```python
from build123d import *

# Parameters (mm, degrees)
F1_DEPTH = 25.4
F3_D     = 3.7973
F3_DEPTH = 101.6
F3_TIP   = 1.1408240143
F4_R     = 2.54


with BuildPart() as f1:
    # F0 (on Front) → F1 (new body)
    with BuildSketch(Plane.XZ):
        with BuildLine():
            ThreePointArc((11.684, 0), (0, -11.684), (-11.684, 0))
            Line((-11.684, 0), (-11.684, 11.684))
            Line((-11.684, 11.684), (-31.75, 11.684))
            Line((-31.75, 11.684), (-31.75, 6.604))
            Line((-31.75, 6.604), (-16.764, 6.604))
            Line((-16.764, 6.604), (-16.764, 0))
            ThreePointArc((-16.764, 0), (0, -16.764), (16.764, 0))
            Line((16.764, 0), (16.764, 6.604))
            Line((16.764, 6.604), (31.75, 6.604))
            Line((31.75, 6.604), (31.75, 11.684))
            Line((31.75, 11.684), (11.684, 11.684))
            Line((11.684, 11.684), (11.684, 0))
        make_face()
    extrude(amount=F1_DEPTH)

    # F3
    with Locations(Plane(origin=(0, 0, 6.604), x_dir=(1, 0, 0), z_dir=(0, 0, -1))):
        with Locations((-25.4, 12.7), (25.4, 12.7)):
            Hole(F3_D / 2, depth=F3_DEPTH)
            with Locations((0, 0, -(F3_DEPTH + F3_TIP / 2))):  # 118° drill point
                Cone(0, F3_D / 2, F3_TIP, mode=Mode.SUBTRACT)

    # F4
    f4_edges = [f1.edges().sort_by_distance(p)[0] for p in [
        (16.764, -12.7, 6.604),
        (-16.764, -12.7, 6.604),
    ]]
    fillet(f4_edges, radius=F4_R)


solid = f1.part
```
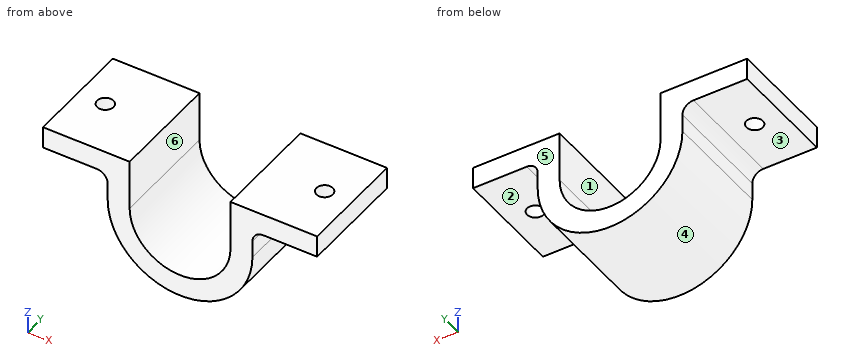
Geometry check sheet. Reference: the model listing, model coordinates, mm. Face numbers are marked on the shaded views. A direction names the side the tool comes from. Give positions to 0.01 mm unless a question says otherwise; leave off trailing zeros. Write each loop counter-clockwise with the first axis right and the second up, starting at its lowest first coordinate (ties: lowest second). Pieces come first, ordered by that corner, then holes. Notation, with made-up numbers: (-10, 83) -> (0, 83) arc R12 ccw to (0, 106) -> close; hole circle Ø4 at (10, 38). An arc over 180 degrees is marked (long way). One line per question, with ' | ' between items.
Item 1: Access from +Z, -Z, +X, -X, +Y, -Y to the whole of each face (thin tool, end or side, straight path). Record for the marked faces 1, 2 and 3.
Determined:
face 1: +Z, +Y, -Y | face 2: -Z, +X, +Y, -Y | face 3: -Z, -X, +Y, -Y
Item 2: Draft check along X on the marked faces 4, 5 and 6. Enter one of: released by +X, released by -X, zero draft, split by the parting line, or undercut.
Determined:
face 4: split by the parting line | face 5: zero draft | face 6: undercut
Item 3: Depth check by flat-ended pin: pin 1 (3.5 mm diameter, centred on x = 25.4, y = -12.7, fed in from +Z); pin 2 (4.5 mm diameter, centred on y = -8, z = 1.5, fed in from +X); pin 3 (5 mm diameter, centred on x = -19.5, y = -13.5, fed in from -Z); pin 4 (3 mm diameter, centred on x = -0.5, y = -6.5, fed in from +Z). Enter the tip coordinate at first touch or a pass-through.
Determined:
pin 1: through | pin 2: x = 16.76 | pin 3: z = 5.13 | pin 4: z = -11.51
Item 4: Sectioned sample at D-D, the plane x = 15. Record the boundary of the cut face in (y, z), plus the area to 3 significant figures.
Determined:
outline: (-25.4, -7.49) -> (0, -7.49) -> (0, 11.68) -> (-25.4, 11.68) -> close | area: 487 mm^2
Item 5: Sectioned sample at C-C, the plane y = -17.25. Record the boundary of the cut face in (x, z), plus the area to 3 significant figures.
Determined:
outline: (-31.75, 6.6) -> (-19.3, 6.6) arc R2.54 cw to (-16.76, 4.06) -> (-16.76, 0) arc R16.76 ccw to (16.76, 0) -> (16.76, 4.06) arc R2.54 cw to (19.3, 6.6) -> (31.75, 6.6) -> (31.75, 11.68) -> (11.68, 11.68) -> (11.68, 0) arc R11.68 cw to (-11.68, 0) -> (-11.68, 11.68) -> (-31.75, 11.68) -> close | area: 501 mm^2
Item 6: Scan lines: line 1 along X through (y, z) = (-12.7, 9.6); line 2 along Y through (x, z) = (25.4, 10.5); line 3 along X through (y, z) = (-17.5, 3). Record each from-to range of solid material in increasing order.
Determined:
line 1: -31.75 to -27.3, -23.5 to -11.68, 11.68 to 23.5, 27.3 to 31.75 | line 2: -25.4 to -14.6, -10.8 to 0 | line 3: -16.76 to -11.68, 11.68 to 16.76
Item 7: Sectioned sample at B-B, the plane y = -12.7. Record the boundary of the cut face in (x, z).
Determined:
outline: (-31.75, 6.6) -> (-27.3, 6.6) -> (-27.3, 11.68) -> (-31.75, 11.68) -> close; (-23.5, 6.6) -> (-19.3, 6.6) arc R2.54 cw to (-16.76, 4.06) -> (-16.76, 0) arc R16.76 ccw to (16.76, 0) -> (16.76, 4.06) arc R2.54 cw to (19.3, 6.6) -> (23.5, 6.6) -> (23.5, 11.68) -> (11.68, 11.68) -> (11.68, 0) arc R11.68 cw to (-11.68, 0) -> (-11.68, 11.68) -> (-23.5, 11.68) -> close; (27.3, 6.6) -> (31.75, 6.6) -> (31.75, 11.68) -> (27.3, 11.68) -> close
Item 8: Sectioned sample at A-A, the plane x = -25.4. Record the boundary of the cut face in (y, z).
Determined:
outline: (-25.4, 6.6) -> (-14.6, 6.6) -> (-14.6, 11.68) -> (-25.4, 11.68) -> close; (-10.8, 6.6) -> (0, 6.6) -> (0, 11.68) -> (-10.8, 11.68) -> close
